```python
from build123d import *

# Parameters (mm, degrees)
F0_W         = 9.75
F0_H         = 9.75
F0_W_2       = 6
F0_H_2       = 6
F1_DEPTH     = 5
F4_W         = 1
F4_H         = 10.4783805975
F5_DEPTH     = 7.5
F6_T4_ANGLE  = 90
F6_T10_ANGLE = 90
F6_T16_ANGLE = 90
F6_T22_ANGLE = 90


# Not quite as in the source:
# - a fillet or chamfer that OpenCascade refuses, or shapes differently, is made with other operations: its cross-section is extruded or revolved along the edge and cut away or added


with BuildPart() as f1:
    # F0 (on Top) → F1 (new body)
    with BuildSketch(Plane.XY):
        Rectangle(F0_W, F0_H)
        Rectangle(F0_W_2, F0_H_2, mode=Mode.SUBTRACT)
    extrude(amount=F1_DEPTH)

    # F2 (on Front) → F3 (revolve)
    with BuildSketch(Plane.XZ):
        with BuildLine():
            Line((3, 25), (3, 5))
            Line((3, 5), (4.5, 5))
            Line((4.5, 5), (4.5, 17.5993331894))
            add(Edge.make_bspline(
                [(3.5845720258, 25), (4.1028451178, 23.9598143656), (5.5548848687, 19.7320627697), (4.5, 17.5993331894)],
                knots=[0, 0, 0, 0, 7.4570689696, 7.4570689696, 7.4570689696, 7.4570689696], degree=3))
            Line((3.5845720258, 25), (3, 25))
        make_face()
    revolve(axis=Axis((0, 0, 5.0040013157), (0, 0, -1)))

    # F4 (on face) → F5 (cut)
    with BuildSketch(Plane.XY.offset(25)):
        with Locations((0, 5.5278654333)):
            Rectangle(F4_W, F4_H)
        Polygon((0, -0.5773502692), (-0.5, 0.2886751346), (-9.574543788, -4.9505151642), (-9.074543788, -5.8165405679), align=None)
        Polygon((0.5, 0.2886751346), (-0.5, 0.2886751346), (0, -0.5773502692), align=None)
        Polygon((9.574543788, -4.9505151642), (0.5, 0.2886751346), (0, -0.5773502692), (9.074543788, -5.8165405679), align=None)
    extrude(amount=-F5_DEPTH, mode=Mode.SUBTRACT)

    # F6: chamfer of 1.24 on 1 edges, made by hand


with BuildPart() as f6_tool2:
    # F6_s3 → F6_t4 (revolve)
    with BuildSketch(Plane.YZ):
        Polygon((-3, 6.24), (-4.24, 5), (-3, 5), align=None)
    revolve(axis=Axis((0, 0, 5), (0, 0, -1)), revolution_arc=F6_T4_ANGLE)

    split(bisect_by=Plane.XZ.offset(3), keep=Keep.BOTTOM)

    split(bisect_by=Plane.YZ.offset(-3), keep=Keep.TOP)


with BuildPart() as f1_1:
    add(f1.part)

    # F6_t1: cut F6_tool2
    add(f6_tool2.part, mode=Mode.SUBTRACT)


with BuildPart() as f6_tool8:
    # F6_s9 → F6_t10 (revolve)
    with BuildSketch(Plane.XZ):
        Polygon((3, 6.24), (4.24, 5), (3, 5), align=None)
    revolve(axis=Axis((0, 0, 5), (0, 0, -1)), revolution_arc=F6_T10_ANGLE)

    split(bisect_by=Plane.YZ.offset(3), keep=Keep.BOTTOM)

    split(bisect_by=Plane.XZ.offset(3), keep=Keep.BOTTOM)


with BuildPart() as f1_2:
    add(f1_1.part)

    # F6_t7: cut F6_tool8
    add(f6_tool8.part, mode=Mode.SUBTRACT)


with BuildPart() as f6_tool14:
    # F6_s15 → F6_t16 (revolve)
    with BuildSketch(Plane.XZ):
        Polygon((-3, 6.24), (-4.24, 5), (-3, 5), align=None)
    revolve(axis=Axis((0, 0, 5), (0, 0, -1)), revolution_arc=F6_T16_ANGLE)

    split(bisect_by=Plane.YZ.offset(-3), keep=Keep.TOP)

    split(bisect_by=Plane.XZ.offset(-3), keep=Keep.TOP)


with BuildPart() as f1_3:
    add(f1_2.part)

    # F6_t13: cut F6_tool14
    add(f6_tool14.part, mode=Mode.SUBTRACT)


with BuildPart() as f6_tool20:
    # F6_s21 → F6_t22 (revolve)
    with BuildSketch(Plane.YZ):
        Polygon((3, 6.24), (4.24, 5), (3, 5), align=None)
    revolve(axis=Axis((0, 0, 5), (0, 0, -1)), revolution_arc=F6_T22_ANGLE)

    split(bisect_by=Plane.YZ.offset(3), keep=Keep.BOTTOM)

    split(bisect_by=Plane.XZ.offset(-3), keep=Keep.TOP)


with BuildPart() as f1_4:
    add(f1_3.part)

    # F6_t19: cut F6_tool20
    add(f6_tool20.part, mode=Mode.SUBTRACT)


solid = f1_4.part
```
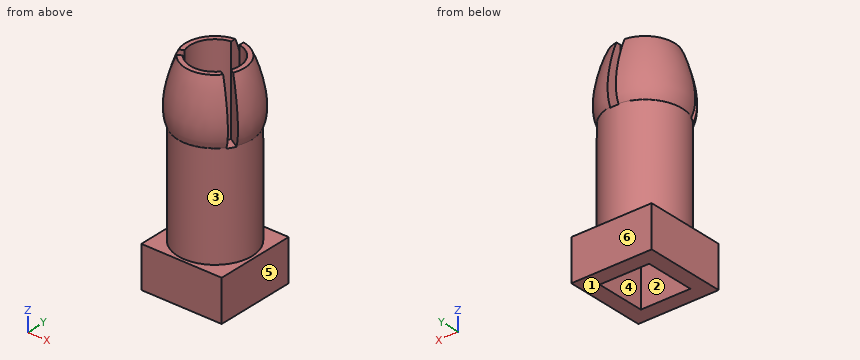
For this review, take the finished solid that the model builds, in its own axes (mm). Face numbers are marked on the shaded views. A direction names the side the tool comes from. Give positions to 0.01 mm unless a question says otherwise; leave off trailing zeros. Write each loop counter-clockwise with the first axis right and the second up, starting at its lowest first coordinate (ties: lowest second). Pieces come first, ordered by that corner, then holes. Notation, with made-up numbers: M -24.5,40 L -20.5,40 A10 cw -20.5,48 Z; hole C 68.25,48 d3. An arc over 180 degrees is marked long. Answer as a JSON object with one key per item and string values. Group by question number.
Item 1: Tool access review of the marked faces 1, 2 and 3: name each direction out of +Z, -Z, +X, -X, +Y, -Y from which nothing blocks a thin tool from reaching the whole face with its end or side.
Item 2: Consider section B-B on z = 23. Count the separate pieces of the cut face and the enclosed holes in it, plus the area to 3 significant figures.
Item 3: Draft analysis for pull direction Y (two halves, no side actions). For the marked faces 4, 5 and 6, state which applies: +Y half, -Y half, draft (parallel to the pull), parting line (faces both ways), or undercut.
Item 4: For pin 1 Ø1 at (x, z) = (-0.5, 11.5) entering from +Y; pin 2 Ø5 at (y, z) = (3, 12) entering from -X; pin 3 Ø1.5 at (y, z) = (3.5, 21) entering from +X; pin 4 Ø3 at (x, y) = (-1.5, -3) entering from -Z, all flat-tipped, find the tip position at first contact; note any pin that passes through.
Item 5: Consider section A-A on z = 4. Write out the cut boundary in (x, y) (3 decimals), plus the area to 3 significant figures.
Item 6: For probe 1 along X at (y, z) = (0, 10.75); probe 2 along Y at (x, z) = (0.5, 3.75) (3 decimals), list the stretches that pass through material, from the lowest coordinate up. Write a range as [from, to].
Item 7: Consider section C-C on z = 10.25. Write out the cut boundary in (x, y), plus the area to 3 significant figures.
Check result:
{
 "1": {"face 1": "-Z, +X, -X, +Y, -Y", "face 2": "-Z", "face 3": "none"},
 "2": {"separate pieces": "3", "enclosed holes": "0", "area": "26.2 mm^2"},
 "3": {"face 4": "undercut", "face 5": "draft", "face 6": "+Y half"},
 "4": {"pin 1": "stops at y = 4.5", "pin 2": "stops at x = -4.47", "pin 3": "stops at x = 3.9", "pin 4": "stops at z = 0"},
 "5": {"outline": "M -4.875,-4.875 L 4.875,-4.875 L 4.875,4.875 L -4.875,4.875 Z; hole M -3,-3 L 3,-3 L 3,3 L -3,3 Z", "area": "59.1 mm^2"},
 "6": {"probe 1": "x = [-4.5, -3], [3, 4.5]", "probe 2": "y = [-4.875, -3], [3, 4.875]"},
 "7": {"outline": "C 0,0 d9; hole C 0,0 d6", "area": "35.3 mm^2"}
}
